Autodesk Inventor part; units mm, degrees
ref_plane "YZ Plane" through (0, 0, 0) normal (1, 0, 0) x (0, 1, 0)
ref_plane "XZ Plane" through (0, 0, 0) normal (0, 1, 0) x (-1, 0, 0)
ref_plane "XY Plane" through (0, 0, 0) normal (0, 0, 1) x (1, 0, 0)
sketch "Sketch1" plane through (0, 0, 0) normal (0, 0, 1) x (1, 0, 0)
  line L0 (-16, -24) -> (16, -24)
  line L1 (16, -24) -> (16, 24)
  line L2 (16, 24) -> (-16, 24)
  line L3 (-16, 24) -> (-16, -24)
  line L4 (-16, -24) -> (16, 24) construction
  line L5 (16, -24) -> (-16, 24) construction
  point P0 (0, 0)
  dimension "d0" = 32
  dimension "d1" = 48
extrude "Extrusion1" add sketch "Sketch1" along normal blind 3.175
sketch "Sketch2" plane through (0, 0, 3.175) normal (0, 0, 1) x (1, 0, 0)
  circle A0 centre (0, -12) radius 5
  line L0 (-16, 24) -> (-16, -24) construction
  line L1 (-16, 0) -> (16, 0) construction
  line L2 (16, -24) -> (16, 24) construction
  circle A1 centre (-6, -6) radius 2
  circle A2 centre (-6, -18) radius 2
  circle A3 centre (6, -18) radius 2
  circle A4 centre (6, -6) radius 2
  circle A5 centre (0, 12) radius 5
  circle A6 centre (-6, 6) radius 2
  circle A7 centre (-6, 18) radius 2
  circle A8 centre (6, 18) radius 2
  circle A9 centre (6, 6) radius 2
  point P0 (0, 0)
  dimension "d4" = 10
  dimension "d5" = 12
  dimension "d6" = 4
  dimension "d7" = 6
  dimension "d8" = 6
  dimension "d11" = 360
extrude "Extrusion2" cut sketch "Sketch2" against normal through all
chamfer "Chamfer1" distance 2 angle 45 4 edges at (16, 24, 1.5875) (-16, 24, 1.5875) (16, -24, 1.5875) (-16, -24, 1.5875)
properties part number "UpperLayerSupportPlate"
Geometry: final body of the model. Coordinates: model frame, mm. Coordinates: 2 decimals unless noted, no trailing zeros. Order: outer loops, then holes, each group sorted by start corner. A loop starts at its lowest first (then second) coordinate and runs counter-clockwise, first axis right, second up. Notation, with made-up numbers: (75.25, 4.5) - (88.25, 4.5) arc R28 cw to (88.25, 28.5) - close; hole circle Ø5 at (9, 56). An arc over 180 degrees is marked (long way). Write each question's results on one line, items separated by ' | '.
(1) Section query A-A, the plane y = -6. Return the cut outline in (x, z) (3 decimals), plus the area to 3 significant figures.
Values found:
outline: (-16, 0) - (-8, 0) - (-8, 3.175) - (-16, 3.175) - close; (-4, 0) - (4, 0) - (4, 3.175) - (-4, 3.175) - close; (8, 0) - (16, 0) - (16, 3.175) - (8, 3.175) - close | area: 76.2 mm²
(2) Line query: line 1 (Y direction, x = 0, z = 1.95); line 2 (Y direction, x = -6, z = 1.9); line 3 (X direction, y = 18.5, z = 1.65). Output: solid intervals per line, ascending. Write a range as [from, to].
Values found:
line 1: y = [-24, -17], [-7, 7], [17, 24] | line 2: y = [-24, -20], [-16, -8], [-4, 4], [8, 16], [20, 24] | line 3: x = [-16, -7.94], [-4.06, 4.06], [7.94, 16]
(3) Section query C-C, the plane z = 2.45. Count the separate pieces of the cut face and the enclosed holes in it, plus the area to 3 significant figures.
Values found:
separate pieces: 1 | enclosed holes: 10 | area: 1,270 mm²
(4) Section query B-B, the plane x = -6. Return the cut outline in (y, z) (3 decimals).
Values found:
outline: (-24, 0) - (-20, 0) - (-20, 3.175) - (-24, 3.175) - close; (-16, 0) - (-8, 0) - (-8, 3.175) - (-16, 3.175) - close; (-4, 0) - (4, 0) - (4, 3.175) - (-4, 3.175) - close; (8, 0) - (16, 0) - (16, 3.175) - (8, 3.175) - close; (20, 0) - (24, 0) - (24, 3.175) - (20, 3.175) - close
(5) First-contact query: pin 1 Ø6 at (x, y) = (0, -12) entering from +Z. Flat tip, straight axial feed; report the tip coordinate or a pass-through.
Values found:
pin 1: passes through
(6) Mould query, pull axis Y, two halves, no side actions, for faces 1 (the face through (0, 24, 2)), 2 (the face through (0, -24, 2)), 3 (the face through (4.526, 7.352, 1.61)). Classes: +Y half, -Y half, draft (parallel to the pull), parting line (faces both ways), or undercut.
Values found:
face 1: +Y half | face 2: -Y half | face 3: undercut
(7) Section query D-D, the plane y = 9. Return the cut outline in (x, z) (3 decimals), plus the area to 3 significant figures.
Values found:
outline: (-16, 0) - (-4, 0) - (-4, 3.175) - (-16, 3.175) - close; (4, 0) - (16, 0) - (16, 3.175) - (4, 3.175) - close | area: 76.2 mm²
